Work out the finished part from the listing and answer in its coordinate system (mm). A direction names the side the tool comes from. Round coordinates to 2 decimals unless told otherwise and drop trailing zeros.
1. A tool of negligible diameter and unlimited length cuts with its end or side. For faces 4 (the face through (-44.03, 1.48, -12.03)), 5 (the face through (-92.115, 1.479, -46.011)), 6 (the face through (-58.883, 1.479, -1.284)), from which of +Z, -Z, +X, -X, +Y, -Y can it reach the whole face along a straight path? Write none if from no direction.
2. Straight lines are drawn through the part: probe 1 along Z at (x, y) = (-8, 1.6); probe 2 along X at (y, z) = (1.6, -51.5); probe 3 along Z at (x, y) = (-65, 1.3). For each, find the intervals that lie inside material, in ascending order.
3. Determine the mould class of faces 1 (the face through (-85.75, 1.48, -24.61)), 2 (the face through (-83.01, 1.48, -39.99)), 3 (the face through (-50.62, 1.52, -13.72)) for opening direction X: pulls with the +X half, pulls with the -X half, needs draft (parallel to the pull), parting line crosses it, or undercut.
4. Flat-ended cylindrical pins translate along their axes: pin 1 Ø0.9 at (x, y) = (-28.5, 1) entering from -Z; pin 2 Ø1.5 at (y, z) = (1.5, -13) entering from -X; pin 3 Ø1.7 at (y, z) = (1.5, -25.5) entering from +X. Find the tip coordinate at first contact, or state that the pin passes through.
```python
from build123d import *

# Parameters (mm, degrees)
BOSS_EXTRUDE1_DEPTH = 3
FILLET1_R           = 1.5


with BuildPart() as part:
    # Sketch1 → Boss-Extrude1 (new body)
    with BuildSketch(Plane(origin=(0, 0, 0), x_dir=(1, 0, 0), z_dir=(0, 1, 0))):
        with BuildLine():
            Line((0, 0), (0, -4.9))
            Line((0, -4.9), (-8.07, -4.9))
            ThreePointArc((-8.07, -4.9), (-12.492074003, -6.540978064), (-16.72, -4.45))
            Line((-16.72, -4.45), (-21.1, -8.34))
            Line((-21.1, -8.34), (-25.391000021, -4.9))
            Line((-25.391000021, -4.9), (-29.72, -8.34))
            Line((-29.72, -8.34), (-32.678148271, -3.564930925))
            Line((-32.678148271, -3.564930925), (-36.614261147, -7.659439528))
            Line((-36.614261147, -7.659439528), (-40.562742989, -2.671583593))
            Line((-40.562742989, -2.671583593), (-45.125314278, -6.1674487))
            Line((-45.125314278, -6.1674487), (-48.772662965, 0.055817603))
            Line((-48.772662965, 0.055817603), (-53.951591598, -3.564930925))
            Line((-53.951591598, -3.564930925), (-55.938419332, 2.377817283))
            Line((-55.938419332, 2.377817283), (-61.936703958, 0.149885503))
            Line((-61.936703958, 0.149885503), (-63.582832138, 5.91))
            Line((-63.582832138, 5.91), (-70.22, 5.91))
            Line((-70.22, 5.91), (-71.604933744, 10.75614566))
            Line((-71.604933744, 10.75614566), (-76.607483243, 11.297362631))
            Line((-76.607483243, 11.297362631), (-77.433672711, 16.398034852))
            Line((-77.433672711, 16.398034852), (-82.492501507, 17.477107174))
            Line((-82.492501507, 17.477107174), (-83.382855617, 23.343000893))
            Line((-83.382855617, 23.343000893), (-88.482100064, 26.076459388))
            Line((-88.482100064, 26.076459388), (-87.341224149, 31.951970353))
            Line((-87.341224149, 31.951970353), (-91.277246058, 35.3745981))
            Line((-91.277246058, 35.3745981), (-89.794107367, 39.253576213))
            Line((-89.794107367, 39.253576213), (-93.730129276, 42.390984981))
            Line((-93.730129276, 42.390984981), (-90.94122884, 48.642955937))
            ThreePointArc((-90.94122884, 48.642955937), (-90.725239113, 54.836582666), (-85.903522924, 50.94316301))
            Line((-85.903522924, 50.94316301), (-87.217276284, 44.958621486))
            Line((-87.217276284, 44.958621486), (-82.368553642, 42.665402728))
            Line((-82.368553642, 42.665402728), (-83.70912889, 37.071165861))
            Line((-83.70912889, 37.071165861), (-78.394556731, 35.535845015))
            Line((-78.394556731, 35.535845015), (-79.175897543, 29.124170033))
            Line((-79.175897543, 29.124170033), (-73.918336593, 27.970006705))
            Line((-73.918336593, 27.970006705), (-73.918336593, 23.343000893))
            Line((-73.918336593, 23.343000893), (-69.072893301, 24.443370455))
            Line((-69.072893301, 24.443370455), (-68.193719482, 20.137924483))
            Line((-68.193719482, 20.137924483), (-63.570641565, 20.736646715))
            Line((-63.570641565, 20.736646715), (-63.025832704, 16.726559775))
            Line((-63.025832704, 16.726559775), (-58.539054065, 19.028863157))
            Line((-58.539054065, 19.028863157), (-56.712577987, 14.764331957))
            Line((-56.712577987, 14.764331957), (-52.617493847, 17.195788166))
            Line((-52.617493847, 17.195788166), (-50.838197485, 13.029757816))
            Line((-50.838197485, 13.029757816), (-46.752937471, 15.232009778))
            Line((-46.752937471, 15.232009778), (-42.029094435, 9.68))
            Line((-42.029094435, 9.68), (-43.497257011, 2.76895697))
            ThreePointArc((-43.497257011, 2.76895697), (-42.341699959, 0.99), (-40.562742989, 2.145557051))
            Line((-40.562742989, 2.145557051), (-39.047121962, 9.28))
            Line((-39.047121962, 9.28), (-34.787121962, 9.28))
            Line((-34.787121962, 9.28), (-34.787121962, 2.79))
            ThreePointArc((-34.787121962, 2.79), (-33.287121962, 1.29), (-31.787121962, 2.79))
            Line((-31.787121962, 2.79), (-31.787121962, 9.28))
            Line((-31.787121962, 9.28), (-27.137121962, 9.28))
            Line((-27.137121962, 9.28), (-26.141480642, 2.534880632))
            ThreePointArc((-26.141480642, 2.534880632), (-24.438519401, 1.27), (-23.173638769, 2.972961241))
            Line((-23.173638769, 2.972961241), (-24.05, 8.91))
            Line((-24.05, 8.91), (0, 12.46))
            Line((0, 12.46), (0, 3))
            Line((0, 3), (-10.82, 3))
            ThreePointArc((-10.82, 3), (-12.32, 1.5), (-10.82, 0))
            Line((-10.82, 0), (0, 0))
        make_face()
    extrude(amount=BOSS_EXTRUDE1_DEPTH)

    # Fillet1
    fillet1_edges = [part.edges().sort_by_distance(p)[0] for p in [
        (-40.562742989, 1.5, 2.671583593),
        (-45.125314278, 1.5, 6.1674487),
        (-48.772662965, 1.5, -0.055817603),
        (-53.951591598, 1.5, 3.564930925),
        (-55.938419332, 1.5, -2.377817283),
        (-61.936703958, 1.5, -0.149885503),
        (-63.582832138, 1.5, -5.91),
        (-70.22, 1.5, -5.91),
        (-71.604933744, 1.5, -10.75614566),
        (-76.607483243, 1.5, -11.297362631),
        (-77.433672711, 1.5, -16.398034852),
        (-82.492501507, 1.5, -17.477107174),
        (-83.382855617, 1.5, -23.343000893),
        (-88.482100064, 1.5, -26.076459388),
        (-87.341224149, 1.5, -31.951970353),
        (-91.277246058, 1.5, -35.3745981),
        (-89.794107367, 1.5, -39.253576213),
        (-93.730129276, 1.5, -42.390984981),
        (-87.217276284, 1.5, -44.958621486),
        (-82.368553642, 1.5, -42.665402728),
        (-83.70912889, 1.5, -37.071165861),
        (-78.394556731, 1.5, -35.535845015),
        (-79.175897543, 1.5, -29.124170033),
        (-73.918336593, 1.5, -27.970006705),
        (-73.918336593, 1.5, -23.343000893),
        (-69.072893301, 1.5, -24.443370455),
        (-68.193719482, 1.5, -20.137924483),
        (-63.570641565, 1.5, -20.736646715),
        (-63.025832704, 1.5, -16.726559775),
        (-58.539054065, 1.5, -19.028863157),
        (-56.712577987, 1.5, -14.764331957),
        (-52.617493847, 1.5, -17.195788166),
        (-50.838197485, 1.5, -13.029757816),
        (-46.752937471, 1.5, -15.232009778),
        (0, 1.5, -12.46),
        (0, 1.5, 4.9),
        (-16.72, 1.5, 4.45),
        (-21.1, 1.5, 8.34),
        (-25.391000021, 1.5, 4.9),
        (-29.72, 1.5, 8.34),
        (-32.678148271, 1.5, 3.564930925),
        (-36.614261147, 1.5, 7.659439528),
    ]]
    fillet(fillet1_edges, radius=FILLET1_R)


solid = part.part
```
Worked answers:
1. face 4: -Z, +Y, -Y
1. face 5: -X, +Y, -Y
1. face 6: +Z, +Y, -Y
2. probe 1: z = -11.28 to -3, 0 to 4.9
2. probe 2: x = -92.75 to -85.83
2. probe 3: z = -20.55 to -5.91
3. face 1: pulls with the -X half
3. face 2: pulls with the +X half
3. face 3: undercut
4. pin 1: stops at z = -9.28
4. pin 2: stops at x = -77
4. pin 3: stops at x = -73.81
